Autodesk Fusion 360 part; units mm, degrees
sketch "Sketch1" plane through (0, 0, 0) normal (0, 1, 0) x (1, 0, 0)
  line L0 (20, 20) -> (-20, 20)
  line L1 (-20, 20) -> (-20, -20)
  line L2 (-20, -20) -> (20, -20)
  line L3 (20, -20) -> (20, 20)
  line L4 (20, 20) -> (-20, -20) construction
  line L5 (-20, 20) -> (20, -20) construction
  dimension "d1" = 40
extrude "Extrude1" add sketch "Sketch1" along normal blind 20
sketch "Sketch2" plane through (0, 20, 0) normal (0, 1, 0) x (-1, 0, 0)
  line L0 (-20, 20) -> (-20, -20)
  line L1 (-20, -20) -> (20, -20)
  line L2 (20, -20) -> (20, 20)
  line L3 (20, 20) -> (-20, 20)
hole "Hole1" at (0, 20, 0) direction (0, -1, 0) diameter 28 end through all
sketch "Sketch3" plane through (0, 0, 20) normal (0, 0, 1) x (1, 0, 0)
  line L0 (-20, 0) -> (20, 0)
  line L1 (20, 0) -> (20, 20)
  line L2 (20, 20) -> (-20, 20)
  line L3 (-20, 20) -> (-20, 0)
  line L4 (2, 4) -> (-2, 4)
  line L5 (-2, 4) -> (-2, -4)
  line L6 (-2, -4) -> (2, -4)
  line L7 (2, -4) -> (2, 4)
  line L8 (2, 4) -> (-2, -4) construction
  line L9 (-2, 4) -> (2, -4) construction
  dimension "d7" = 4
  dimension "d8" = 8
extrude "Extrude2" cut sketch "Sketch3" against normal blind 10 contours L0 L4 L5 L7
sketch "Sketch4" plane through (0, 0, 0) normal (0, -1, 0) x (1, 0, 0)
  line L0 (-2, 13.8564) -> (-2, 20)
  line L1 (-2, 20) -> (-20, 20)
  line L2 (-20, 20) -> (-20, -20)
  line L3 (-20, -20) -> (20, -20)
  line L4 (20, -20) -> (20, 20)
  line L5 (20, 20) -> (2, 20)
  line L6 (2, 20) -> (2, 13.8564)
  arc A0 (-2, 13.8564) -> (2, 13.8564) centre (0, 0) ccw
  line L7 (25, -12) -> (5, -12)
  line L8 (5, -12) -> (5, 12)
  line L9 (5, 12) -> (25, 12)
  line L10 (25, 12) -> (25, -12)
  line L11 (25, -12) -> (5, 12) construction
  line L12 (5, -12) -> (25, 12) construction
  point P0 (15, 0)
extrude "Extrude3" cut sketch "Sketch4" against normal blind 6 contours L4 A0 L7 L9
sketch "Sketch5" plane through (0, 0, 0) normal (0, -1, 0) x (1, 0, 0)
  line L0 (20, -12) -> (7.2111, -12)
  arc A0 (-2, 13.8564) -> (7.2111, -12) centre (0, 0) ccw
  line L1 (-2, 13.8564) -> (-2, 20)
  line L2 (-2, 20) -> (-20, 20)
  line L3 (-20, 20) -> (-20, -20)
  line L4 (-20, -20) -> (20, -20)
  line L5 (20, -20) -> (20, -12)
  line L6 (12, -9) -> (-12, -9)
  line L7 (-12, -9) -> (-12, -31)
  line L8 (-12, -31) -> (12, -31)
  line L9 (12, -31) -> (12, -9)
  line L10 (12, -9) -> (-12, -31) construction
  line L11 (-12, -9) -> (12, -31) construction
  point P0 (0, -20)
extrude "Extrude4" cut sketch "Sketch5" against normal blind 6 contours L0 A0 L4 L6 L7 L9
sketch "Sketch6" plane through (0, 0, 0) normal (0, -1, 0) x (1, 0, 0)
  line L0 (-12, -20) -> (-12, -9)
  line L1 (-12, -9) -> (-10.7238, -9)
  arc A0 (-2, 13.8564) -> (-10.7238, -9) centre (0, 0) ccw
  line L2 (-2, 13.8564) -> (-2, 20)
  line L3 (-2, 20) -> (-20, 20)
  line L4 (-20, 20) -> (-20, -20)
  line L5 (-20, -20) -> (-12, -20)
  line L6 (-4, 12) -> (-36, 12)
  line L7 (-36, 12) -> (-36, -12)
  line L8 (-36, -12) -> (-4, -12)
  line L9 (-4, -12) -> (-4, 12)
  line L10 (-4, 12) -> (-36, -12) construction
  line L11 (-36, 12) -> (-4, -12) construction
  point P0 (-20, 0)
extrude "Extrude5" cut sketch "Sketch6" against normal blind 6 contours L0 L1 A0 L4 L6 L8
Source: CAD feature listing. Evaluate the final solid. Frame: model axes, mm. A direction names the side the tool comes from. Give positions to 0.01 mm unless a question says otherwise; leave off trailing zeros. Order: outer loops, then holes, each group sorted by start corner. A loop starts at its lowest first (then second) coordinate and runs counter-clockwise, first axis right, second up. Notation, with made-up numbers: (14, 48.5) -> (51, 48.5) arc R33 cw to (51, 76.5) -> close; hole circle Ø2 at (-15.75, 52.25). An arc over 180 degrees is marked (long way). Write item = value, one per line.
Q1. Cut plane C-C, the plane y = 5. Output: boundary loops of the cut face in (x, z).
Data:
outline = (-20, -20) -> (-12, -20) -> (-12, -12) -> (-20, -12) -> close; (-20, 12) -> (-7.21, 12) arc R14 cw to (7.21, 12) -> (20, 12) -> (20, 20) -> (-20, 20) -> close; (12, -20) -> (20, -20) -> (20, -12) -> (12, -12) -> close
Q2. Material intervals for line 1 (Z direction, x = -0.5, y = 16.25); line 2 (X direction, y = 12, z = 0); line 3 (Y direction, x = -14.5, z = -3.5), sorted ascending. Write a range as from..to.
Data:
line_1 = -20..-13.99, 13.99..20
line_2 = -20..-14, 14..20
line_3 = 6..20
Q3. Cut plane B-B, the plane x = 0. Output: boundary loops of the cut face in (y, z), and give its area (3 significant figures).
Data:
outline = (4, 14) -> (20, 14) -> (20, 20) -> (4, 20) -> close; (6, -20) -> (20, -20) -> (20, -14) -> (6, -14) -> close
area = 180 mm^2
Q4. Cut plane A-A, the plane z = 0. Output: boundary loops of the cut face in (x, y), and give its area (3 significant figures).
Data:
outline = (-20, 6) -> (-14, 6) -> (-14, 20) -> (-20, 20) -> close; (14, 6) -> (20, 6) -> (20, 20) -> (14, 20) -> close
area = 168 mm^2
Q5. Pin query (flat end, axial travel): pin 1 (1.2 mm diameter, centred on x = 0, z = 17.5, fed in from -Y); pin 2 (3 mm diameter, centred on x = 15, z = 1, fed in from -Y). Return the tip coordinate at first contact, or that it passes through.
Data:
pin_1 = 4
pin_2 = 6
Q6. Cut plane D-D, the plane y = 13.25. Output: boundary loops of the cut face in (x, z), and give its area (3 significant figures).
Data:
outline = (-20, -20) -> (20, -20) -> (20, 20) -> (-20, 20) -> close; hole circle Ø28 at (0, 0)
area = 984 mm^2
Q7. Set-up query: faces 1 (the face through (-14, 3, 12)), 2 (the face through (-12, 3, -16)), 3 (the face through (0, 4, 17)). Return all of +Z, -Z, +X, -X, +Y, -Y with unobstructed straight access to the full face (end or side cutting, diameter ignored); none if empty.
Data:
face_1 = +X, -X, -Y
face_2 = -Z, -Y
face_3 = +Z, -Z, -Y
Q8. Pull-direction query (Z, two-part tool) for faces 4 (the face through (-11, 0, 16)), 5 (the face through (14, 3, 12)), 6 (the face through (0, 10, 20)); classes: released by +Z, released by -Z, zero draft, split by the parting line, or undercut.
Data:
face_4 = zero draft
face_5 = undercut
face_6 = released by +Z
